```python
from build123d import *

# Parameters (mm, degrees)
BOSS_EXTRUDE1_DEPTH  = 6
SKETCH1_3_R          = 2.5
BOSS_EXTRUDE2_DEPTH  = 6
SKETCH1_5_R          = 5
BOSS_EXTRUDE3_DEPTH  = 6
CUT_EXTRUDE3_DEPTH   = 3
CUT_SWEEP5_PROFILE_R = 1.5
SKETCH1_7_R          = 2.5
BOSS_EXTRUDE4_DEPTH  = 6
CHAMFER1_SIZE        = 1
CUT_EXTRUDE4_DEPTH   = 4


with BuildPart() as part:
    # Sketch1 → Boss-Extrude1 (new body, symmetric)
    with BuildSketch(Plane.XY):
        with BuildLine():
            Line((10.625, 4.960783708), (-9.0625, 7.441175562))
            ThreePointArc((-9.0625, 7.441175562), (-2.514267184, 0.462389669), (-8.153846154, -7.269230769))
            Line((-8.153846154, -7.269230769), (10, -5))
            ThreePointArc((10, -5), (5.009813704, 0.313114563), (10.625, 4.960783708))
        make_face()
    extrude(amount=BOSS_EXTRUDE1_DEPTH, both=True)

    # Sketch1_3 → Boss-Extrude2 (add, symmetric)
    with BuildSketch(Plane.XY):
        with BuildLine():
            ThreePointArc((-8.153846154, -7.269230769), (-2.514267184, 0.462389669), (-9.0625, 7.441175562))
            ThreePointArc((-9.0625, 7.441175562), (-9.530328156, 7.485279444), (-10, 7.5))
            Line((-10, 7.5), (-16.5, 7.5))
            ThreePointArc((-16.5, 7.5), (-17.207106781, 7.207106781), (-17.5, 6.5))
            Line((-17.5, 6.5), (-17.5, 0))
            ThreePointArc((-17.5, 0), (-15.303300859, -5.303300859), (-10, -7.5))
            Line((-10, -7.5), (-8.153846154, -7.269230769))
        make_face()
        with Locations((-10, 0)):
            Circle(SKETCH1_3_R, mode=Mode.SUBTRACT)
    extrude(amount=BOSS_EXTRUDE2_DEPTH, both=True)

    # Sketch1_5 → Boss-Extrude3 (add, symmetric)
    with BuildSketch(Plane.XY):
        with Locations((10, 0)):
            Circle(SKETCH1_5_R)
    extrude(amount=BOSS_EXTRUDE3_DEPTH, both=True)

    # Sketch2 → Cut-Extrude3 (cut, symmetric)
    with BuildSketch(Plane.XY):
        with BuildLine():
            Line((-2, 0), (-2, -8))
            Line((-2, -8), (-10, -8))
            ThreePointArc((-10, -8), (-15.656854249, -5.656854249), (-18, 0))
            Line((-18, 0), (-18, 8.108199506))
            Line((-18, 8.108199506), (-10, 8))
            ThreePointArc((-10, 8), (-4.343145751, 5.656854249), (-2, 0))
        make_face()
    extrude(amount=CUT_EXTRUDE3_DEPTH, both=True, mode=Mode.SUBTRACT)

    # Cut-Sweep5: sweep along a path in Sketch3
    with BuildLine(Plane.XY) as cut_sweep5_path:
        Line((-1.5, 8.191992315), (-1.5, 6.48839012))
        Line((-1.5, 6.48839012), (-1.5, 5))
        ThreePointArc((-1.5, 5), (-0.621320344, 2.878679656), (1.5, 2))
        Line((1.5, 2), (3.5, 2))
        ThreePointArc((3.5, 2), (5.621320344, 2.878679656), (6.5, 5))
        Line((6.5, 5), (6.5, 5.480484859))
        Line((6.5, 5.480484859), (6.5, 8.191992315))
    # Cut-Sweep5 profile (on start of the path) → Cut-Sweep5 (sweep, cut)
    with BuildSketch(Plane(origin=(-1.5, 8.191992315, 0), x_dir=(0, 0, -1), z_dir=(0, -1, 0))):
        Circle(CUT_SWEEP5_PROFILE_R)
    cut_sweep5 = sweep(path=cut_sweep5_path.line, mode=Mode.SUBTRACT)

    # Mirror4: Cut-Sweep5 across plane
    add(cut_sweep5.mirror(Plane.ZX), mode=Mode.SUBTRACT)

    # Sketch1_7 → Boss-Extrude4 (add, symmetric)
    with BuildSketch(Plane.XY):
        with Locations((-10, 0)):
            Circle(SKETCH1_7_R)
    extrude(amount=BOSS_EXTRUDE4_DEPTH, both=True)

    # Chamfer1
    chamfer1_edges = [part.edges().sort_by_distance(p)[0] for p in [
        (-12.5, 0, 3),
        (-12.5, 0, -3),
    ]]
    chamfer(chamfer1_edges, length=CHAMFER1_SIZE)

    # Sketch130 → Cut-Extrude4 (cut, symmetric)
    with BuildSketch(Plane(origin=(0, 0, 0), x_dir=(1, 0, 0), z_dir=(0, 1, 0))):
        Polygon((0, -6), (0, -4), (3, -4), (4, -6), (4, -8.476045259), (0, -8.476045259), align=None)
    cut_extrude4 = extrude(amount=CUT_EXTRUDE4_DEPTH, both=True, mode=Mode.SUBTRACT)

    # Mirror5: Cut-Extrude4 across plane
    add(cut_extrude4.mirror(Plane.XY), mode=Mode.SUBTRACT)


solid = part.part
```
Geometry: final body of the model. Coordinates: model frame, mm. A direction names the side the tool comes from. Coordinates: 2 decimals unless noted, no trailing zeros. Order: outer loops, then holes, each group sorted by start corner. A loop starts at its lowest first (then second) coordinate and runs counter-clockwise, first axis right, second up. Notation, with made-up numbers: M 78.5,-5.75 L 119.5,-5.75 A22 ccw 119.5,15.25 Z; hole C 9.5,-7 d7. An arc over 180 degrees is marked long. Answer as CSV lines item,"result".
Q1. Set-up query: faces 4 (the flat face through (-2, -1.8, 0)), 5 (the flat face through (2, 4, 5)), 6 (the flat face through (2, -4, -5)), 7 (the flat face through (-6, 0, -3)). Return all of +Z, -Z, +X, -X, +Y, -Y with unobstructed straight access to the full face (end or side cutting, diameter ignored); none if empty.
Answers:
face 4,"-Y"
face 5,"+Z"
face 6,"-Z"
face 7,"none"
Q2. Line query: probe 1 along Z at (x, y) = (2.2, -2); probe 2 along Z at (x, y) = (-1.5, -5.45); probe 3 along Y at (x, z) = (2.8, 0). Output: solid intervals per line, ascending. Write a range as [from, to].
Answers:
probe 1,"z = [-4, -1.5], [1.5, 4]"
probe 2,"z = [-6, -1.5], [1.5, 6]"
probe 3,"y = [-5.9, -3.5], [-0.5, 0.5], [3.5, 5.95]"
Q3. Section B-B on z = -0.25. Return the cut outline in (x, y) (3 decimals), and give its area (3 significant figures).
Answers:
outline,"C -10,0 d5; M -6.3,7.093 A8 cw -2,0 L -2,-2.205 A4.479 cw 1.5,-0.521 L 3.5,-0.521 A4.479 cw 7.979,-5 L 7.979,-5.253 L 10,-5 A5 ccw 10.625,4.961 L 7.979,5.294 L 7.979,5 A4.479 cw 3.5,0.521 L 1.5,0.521 A4.479 cw -2.979,5 L -2.979,6.675 Z; M -0.021,-6.253 L 5.021,-5.622 L 5.021,-5 A1.521 ccw 3.5,-3.479 L 1.5,-3.479 A1.521 ccw -0.021,-5 Z; M -0.021,5 A1.521 ccw 1.5,3.479 L 3.5,3.479 A1.521 ccw 5.021,5 L 5.021,5.667 L -0.021,6.302 Z"
area,"129 mm^2"
Q4. Draft query along Y for faces 1 (the cylindrical face through (-3.19, 4.2, 0.04)), 2 (the flat face through (0, 0, -5)), 3 (the flat face through (-6, 0, 3)). Return one class per face: pulls with the +Y half, pulls with the -Y half, needs draft (parallel to the pull), parting line crosses it, or undercut.
Answers:
face 1,"pulls with the -Y half"
face 2,"undercut"
face 3,"needs draft"
Q5. Section D-D on y = 2. Count the separate pieces of the cut face and the enclosed holes in it, and give its area (3 significant figures).
Answers:
separate pieces,"1"
enclosed holes,"2"
area,"277 mm^2"
Q6. First-contact query: P1, Ø2, axis at x = 3, z = 5, coming from the -Y side; P2, Ø3, axis at x = 0, z = -3, coming from the +Y side; P3, Ø1, axis at x = 1.5, z = -5.5, coming from the +Y side. Flat tips, straight axial feed; report the tip coordinate or a pass-through.
Answers:
P1,"stops at y = -6"
P2,"stops at y = 6.49"
P3,"stops at y = 6.17"
Q7. Section C-C on z = 5.25. Return the cut outline in (x, y) (1 decimal).
Answers:
outline,"M -17.5,0 A7.5 ccw -10,-7.5 L 10,-5 A5 ccw 10.6,5 L -9.1,7.4 A7.5 ccw -10,7.5 L -16.5,7.5 A1 ccw -17.5,6.5 Z; hole M 0,-4 L 3.6,-4 L 3.6,4 L 0,4 Z"
Q8. Section A-A on z = -2.5. Return the cut outline in (x, y) (3 decimals), and give its area (3 significant figures).
Answers:
outline,"C -10,0 d6; M -6.3,7.093 A8 cw -2,0 L -2,-6.5 L 10,-5 A5 ccw 10.625,4.961 Z"
area,"214 mm^2"
